from build123d import *

# Parameters (mm, degrees)
SKETCH1_W           = 32
SKETCH1_H           = 44.45
BOSS_EXTRUDE1_DEPTH = 50.8
SKETCH2_W           = 35.808
SKETCH2_H           = 33.016
CUT_EXTRUDE1_DEPTH  = 32
CUT_EXTRUDE2_REACH  = 71.372
SKETCH4_W           = 8.642
SKETCH4_H           = 44.45
CUT_EXTRUDE3_DEPTH  = 65.020236059
SKETCH6_W           = 25.908
SKETCH6_H           = 6.858
CUT_EXTRUDE4_DEPTH  = 5.842
CUT_EXTRUDE5_START  = -44.45
SKETCH7_R           = 1.3
CUT_EXTRUDE5_DEPTH  = 44.45
SKETCH8_W           = 19.3
SKETCH8_H           = 19.05
CUT_EXTRUDE6_DEPTH  = 45.328667801


with BuildPart() as part:
    # Sketch1 → Boss-Extrude1 (new body)
    with BuildSketch(Plane.XY):
        Rectangle(SKETCH1_W, SKETCH1_H)
    extrude(amount=-BOSS_EXTRUDE1_DEPTH)

    # Sketch2 → Cut-Extrude1 (cut)
    with BuildSketch(Plane(origin=(16, 0, 0), x_dir=(0, 0, -1), z_dir=(1, 0, 0))):
        with Locations((17.904, 0)):
            Rectangle(SKETCH2_W, SKETCH2_H)
    extrude(amount=-CUT_EXTRUDE1_DEPTH, mode=Mode.SUBTRACT)

    # Cut-Extrude2: up to this face of the body (flat: up to its plane)
    cut_extrude2_end = Plane(part.part.faces().sort_by_distance((0, -22.225, -25.4))[0])
    # Sketch3 → Cut-Extrude2 (cut, up to the picked face)
    with BuildSketch(Plane(origin=(0, 22.225, 0), x_dir=(1, 0, 0), z_dir=(0, 1, 0)), mode=Mode.PRIVATE) as cut_extrude2_sk1:
        Polygon((-10.508, 7.3), (-10.508, 29.808), (10.508, 29.808), (10.508, 7.3), (16, 7.3), (16, 0), (-16, 0), (-16, 7.3), align=None)
    cut_extrude2_tool1 = split(extrude(cut_extrude2_sk1.sketch, amount=-CUT_EXTRUDE2_REACH, mode=Mode.PRIVATE), bisect_by=cut_extrude2_end, keep=Keep.BOTH, mode=Mode.PRIVATE)
    add(cut_extrude2_tool1.solids().sort_by(Axis((0, 22.225, -13.626975), (0, -1, 0)))[0], mode=Mode.SUBTRACT)

    # Sketch4 → Cut-Extrude3 (cut, through all)
    with BuildSketch(Plane.ZY.offset(16)):
        with Locations((-46.479, 0)):
            Rectangle(SKETCH4_W, SKETCH4_H)
    extrude(amount=-CUT_EXTRUDE3_DEPTH, mode=Mode.SUBTRACT)

    # Sketch6 → Cut-Extrude4 (cut)
    with BuildSketch(Plane(origin=(0, 22.225, 0), x_dir=(1, 0, 0), z_dir=(0, 1, 0))):
        with Locations((0, 35.771215189)):
            Rectangle(SKETCH6_W, SKETCH6_H)
    extrude(amount=-CUT_EXTRUDE4_DEPTH, mode=Mode.SUBTRACT)

    # Sketch7 → Cut-Extrude5 (cut)
    with BuildSketch(Plane(origin=(0, 22.225, 0), x_dir=(1, 0, 0), z_dir=(0, 1, 0)).offset(CUT_EXTRUDE5_START)):
        with Locations(Location((-13.5, 11.808, 0), (0, 0, 270))):
            Circle(SKETCH7_R)
        with Locations(Location((-13.5, 19.808, 0), (0, 0, 270))):
            Circle(SKETCH7_R)
        with Locations(Location((-13.5, 27.808, 0), (0, 0, 270))):
            Circle(SKETCH7_R)
        with Locations(Location((13.5, 27.808, 0), (0, 0, 270))):
            Circle(SKETCH7_R)
        with Locations(Location((13.5, 19.808, 0), (0, 0, 270))):
            Circle(SKETCH7_R)
        with Locations(Location((13.5, 11.808, 0), (0, 0, 270))):
            Circle(SKETCH7_R)
    extrude(amount=CUT_EXTRUDE5_DEPTH, mode=Mode.SUBTRACT)

    # Sketch8 → Cut-Extrude6 (cut, through all)
    with BuildSketch(Plane(origin=(0, 0, -42.158), x_dir=(-1, 0, 0), z_dir=(0, 0, -1))):
        Rectangle(SKETCH8_W, SKETCH8_H)
    extrude(amount=-CUT_EXTRUDE6_DEPTH, mode=Mode.SUBTRACT)


solid = part.part
Model file for the job. Use its own axes, mm. A direction names the side the tool comes from. Give positions to 0.01 mm unless a question says otherwise; leave off trailing zeros. Loops run counter-clockwise (first coordinate to the right, second up) from the corner with the lowest first, then second, coordinate; pieces in that order, holes last.
Item 1: Drop flat-ended pins along their axis: P1, Ø2.5, axis at x = -6, z = -37, coming from the +Y side; P2, Ø10, axis at x = 6.5, y = 3.5, coming from the +Z side; P3, Ø2.5, axis at x = 13.5, z = -11.808, coming from the +Y side. Give the stop position or say it passes through.
Check values:
P1: stops at y = 16.38
P2: stops at z = -35.81
P3: passes through
Item 2: Slice it at B-B (y = -5). Write the cut outline in (x, z), plus the area to 3 significant figures.
Check values:
outline: (-16, -42.16) - (-9.65, -42.16) - (-9.65, -35.81) - (-16, -35.81) - close; (9.65, -42.16) - (16, -42.16) - (16, -35.81) - (9.65, -35.81) - close
area: 80.6 mm2
Item 3: Slice it at D-D (x = 9). Write the cut outline in (y, z) (3 decimals).
Check values:
outline: (-22.225, -42.158) - (-9.525, -42.158) - (-9.525, -35.808) - (-16.508, -35.808) - (-16.508, -29.808) - (-22.225, -29.808) - close; (9.525, -42.158) - (22.225, -42.158) - (22.225, -39.2) - (16.383, -39.2) - (16.383, -35.808) - (9.525, -35.808) - close; (16.508, -32.342) - (22.225, -32.342) - (22.225, -29.808) - (16.508, -29.808) - close
Item 4: Drill centre lines: line 1 along Y through (x, z) = (13, -14) (3 decimals); line 2 along Z through (x, y) = (13.5, -21.1); line 3 along Z through (x, y) = (-5.5, 17.5). Where is each one in solid material? Low to high.
Check values:
line 1: y = -22.225 to -16.508, 16.508 to 22.225
line 2: z = -42.16 to -29.11, -26.51 to -21.11, -18.51 to -13.11, -10.51 to -7.3
line 3: z = -42.16 to -39.2, -32.34 to -29.81
Item 5: Mould opens along Y. For faces 1 (the face through (14.79, 19.33, -19.98)), 2 (the face through (-9.65, 0, -39)), 3 (the face through (4, -16.508, -31)) say: +Y half, -Y half, draft (parallel to the pull), parting line (faces both ways), or undercut.
Check values:
face 1: draft
face 2: undercut
face 3: undercut
Item 6: Which spindle directions (+Z, -Z, +X, -X, +Y, -Y) get a long thin tool onto all of the face, cutting with end or side? Do faces 4 (the face through (9.65, 0, -39)), 5 (the face through (-12.954, 19, -36)), 6 (the face through (10.508, 19, -19)), 7 (the face through (14.79, 19.33, -11.98)). Say none if no direction does.
Check values:
face 4: +Z, -Z
face 5: +Y
face 6: +Z, +Y, -Y
face 7: +Y, -Y
Item 7: Slice it at C-C (y = 17.5). Write the cut outline in (x, z), plus the area to 3 significant figures.
Check values:
outline: (-16, -42.16) - (16, -42.16) - (16, -7.3) - (10.51, -7.3) - (10.51, -29.81) - (-10.51, -29.81) - (-10.51, -7.3) - (-16, -7.3) - close; hole circle Ø2.6 at (-13.5, -27.81); hole circle Ø2.6 at (-13.5, -19.81); hole circle Ø2.6 at (-13.5, -11.81); hole (-12.95, -39.2) - (12.95, -39.2) - (12.95, -32.34) - (-12.95, -32.34) - close; hole circle Ø2.6 at (13.5, -27.81); hole circle Ø2.6 at (13.5, -19.81); hole circle Ø2.6 at (13.5, -11.81)
area: 433 mm2
Item 8: Slice it at A-A (x = -13.5). Give the number of separate pieces and of enclosed holes in the cut face, plus the area to 3 significant figures.
Check values:
separate pieces: 7
enclosed holes: 0
area: 519 mm2
